Read the model definition and answer for the solid it produces. Units are mm, in the model's axes. A direction names the side the tool comes from. Coordinates: 2 decimals unless noted, no trailing zeros. Order: outer loops, then holes, each group sorted by start corner. A loop starts at its lowest first (then second) coordinate and runs counter-clockwise, first axis right, second up. Notation, with made-up numbers: M 74.5,-37 L 102.5,-37 A20 cw 102.5,-10 Z; hole C 62,49 d11. An arc over 180 degrees is marked long. Use a Markdown table: item, result. Add a question column.
1) This flat-tipped pin is pushed along its axis until it touches: pin 1 Ø1.5 at (y, z) = (-28, 5.5) entering from -X. Where does it stop, or does it pass through?
2) Find the intervals of material crossed by probe 1 along X at (y, z) = (-11.5, 2.75); probe 2 along Y at (x, z) = (-0.5, 3.5); probe 3 along X at (y, z) = (-66.5, 1.5), in increasing order. Write a range as [from, to].
3) For faces 1 (the face through (-8.381, -61.483, 5.697)), 2 (the face through (39, -35, 0)), determine the directions among +Z, -Z, +X, -X, +Y, -Y from which every point of the face is accessible in a straight line to the end or side of a thin tool.
4) Find section A-A on y = -49. Write down the section's boundary in (x, z).
from build123d import *

# Parameters (mm, degrees)
SKETCH1_W           = 80
SKETCH1_H           = 71.597374179
BOSS_EXTRUDE1_DEPTH = 10
SKETCH2_R           = 3.909711409
BOSS_EXTRUDE2_DEPTH = 20
FILLET1_R           = 3


with BuildPart() as part:
    # Sketch1 → Boss-Extrude1 (new body)
    with BuildSketch(Plane.XY):
        with Locations((40, -35.798687089)):
            Rectangle(SKETCH1_W, SKETCH1_H)
    extrude(amount=BOSS_EXTRUDE1_DEPTH)

    # Sketch2 → Boss-Extrude2 (add)
    with BuildSketch(Plane.ZY):
        with Locations(Location((4.849229458, -65.299456518, 0), (0, 0, 180))):
            Circle(SKETCH2_R)
    extrude(amount=BOSS_EXTRUDE2_DEPTH)

    # Fillet1
    fillet1_edges = [part.edges().sort_by_distance(p)[0] for p in [
        (-20, -65.299456518, 8.758940867),
    ]]
    fillet(fillet1_edges, radius=FILLET1_R)


solid = part.part
Check result:
| question | item | result |
|---|---|---|
| 1 | pin 1 | stops at x = 0 |
| 2 | probe 1 | x = [0, 80] |
| 2 | probe 2 | y = [-68.97, -61.63] |
| 2 | probe 3 | x = [-18.41, 80] |
| 3 | face 1 | -X |
| 3 | face 2 | -Z, +X, -X, +Y, -Y |
| 4 | outline | M 0,0 L 80,0 L 80,10 L 0,10 Z |
